Verification items for the finished model (mm, model axes). Face numbers are marked on the shaded views. A direction names the side the tool comes from. Round coordinates to 2 decimals unless told otherwise and drop trailing zeros. Write each loop counter-clockwise with the first axis right and the second up, starting at its lowest first coordinate (ties: lowest second). Pieces come first, ordered by that corner, then holes. Notation, with made-up numbers: (-39, 2) - (-29, 2) arc R10 cw to (-29, 9) - close; hole circle Ø9 at (3, -22.5). An arc over 180 degrees is marked (long way). Answer as a JSON object with one key per item and string values.
Autodesk Inventor part; units mm, degrees
ref_plane "YZ Plane" through (0, 0, 0) normal (1, 0, 0) x (0, 1, 0)
ref_plane "XZ Plane" through (0, 0, 0) normal (0, 1, 0) x (-1, 0, 0)
ref_plane "XY Plane" through (0, 0, 0) normal (0, 0, 1) x (1, 0, 0)
sketch "Sketch1" plane through (0, 0, 0) normal (0, 0, 1) x (1, 0, 0)
  line L0 (-32.1306, 17.7406) -> (444.1194, 17.7406)
  line L1 (444.1194, 17.7406) -> (444.1194, -33.0594)
  line L2 (444.1194, -33.0594) -> (-32.1306, -33.0594)
  line L3 (-32.1306, -33.0594) -> (-32.1306, 17.7406)
  point P0 (0, 0)
  dimension "d0" = 476.25
  dimension "d1" = 50.8
extrude "Extrusion1" add sketch "Sketch1" along normal blind 139.7
sketch "Sketch2" plane through (-32.1306, 17.7406, 0) normal (0, 1, 0) x (1, 0, 0)
  line L0 (0, -139.7) -> (476.25, -139.7)
  line L1 (0, 0) -> (476.25, 0)
  line L2 (0, 0) -> (0, -139.7)
  circle A0 centre (75.1417, -80.645) radius 55.88
  circle A1 centre (225.4419, -80.645) radius 55.88
  circle A2 centre (375.7337, -80.645) radius 55.88
  line L3 (150.2833, 0) -> (150.2833, -139.7)
  line L4 (300.5751, 0) -> (300.5751, -139.7)
  line L5 (450.8669, 0) -> (450.8669, -139.7)
  arc A3 (131.0217, -80.645) -> (150.2833, -114.7129) centre (183.3802, -73.521) ccw
  arc A4 (150.2833, -114.7129) -> (169.5619, -80.645) centre (117.2054, -73.5058) ccw
  arc A5 (281.208, -77.0792) -> (300.5751, -114.6812) centre (333.9413, -73.7073) ccw
  arc A6 (300.5751, -114.6812) -> (319.9683, -77.068) centre (267.2357, -73.6855) ccw
  arc A7 (0, -114.6812) -> (19.2617, -80.645) centre (-33.0921, -73.4855) ccw
  arc A8 (431.6137, -80.645) -> (450.8669, -113.4262) centre (483.7537, -72.0665) ccw
  line L6 (450.8669, 0) -> (476.25, 0)
  line L7 (476.25, 0) -> (476.25, -139.7)
  line L8 (476.25, -139.7) -> (450.8669, -139.7)
  line L9 (450.8669, -139.7) -> (450.8669, 0)
  point P0 (32.1306, 0)
  dimension "d4" = 111.76
  dimension "d5" = 111.76
  dimension "d6" = 111.76
  dimension "d7" = 150.2833
  dimension "d8" = 150.2918
  dimension "d9" = 150.2918
  dimension "d10" = 75.1417
  dimension "d11" = 75.1332
  dimension "d12" = 75.1332
  dimension "d13" = 59.055
extrude "Extrusion2" cut sketch "Sketch2" against normal blind 139.7 contours L2 A7 A0 A3 L3 L0 | L3 A4 A1 A5 L4 L0 | L4 A6 A2 A8 L5 L0 | A0 | L5 L1 L7 L0 | A1 | A2
fillet "Fillet1" radius 2.54 1 edges at (418.7363, -7.6594, 113.4262)
fillet "Fillet2" radius 2.54 1 edges at (268.4445, -7.6594, 114.6812)
fillet "Fillet3" radius 2.54 1 edges at (118.1527, -7.6594, 114.7129)
fillet "Fillet4" radius 2.54 1 edges at (-32.1306, -7.6594, 114.6812)
sketch "Sketch3" plane through (-32.1306, 17.7406, 0) normal (0, 1, 0) x (1, 0, 0)
  arc A0 (148.6129, -113.313) -> (151.9544, -113.3138) centre (150.2841, -111.4003) ccw
  arc A1 (298.8914, -113.2506) -> (302.2598, -113.2517) centre (300.5762, -111.3498) ccw
  line L0 (0, 0) -> (450.8669, 0)
  line L1 (37.0382, 0) -> (113.2382, 0)
  line L2 (113.2382, 0) -> (113.2382, -50.8)
  line L3 (113.2382, -50.8) -> (37.0382, -50.8)
  line L4 (37.0382, -50.8) -> (37.0382, 0)
  line L5 (150.2841, -111.4003) -> (150.2841, 5.0811)
  line L6 (263.53, 0) -> (187.33, 0)
  line L7 (187.33, 0) -> (187.33, -50.8)
  line L8 (187.33, -50.8) -> (263.53, -50.8)
  line L9 (263.53, -50.8) -> (263.53, 0)
  line L10 (75.1382, -50.8) -> (75.1382, 0)
  line L11 (300.5762, -111.3498) -> (300.5762, 0)
  line L12 (337.6224, -50.8) -> (337.6224, 0)
  line L13 (337.6224, 0) -> (413.8224, 0)
  line L14 (413.8224, 0) -> (413.8224, -50.8)
  line L15 (413.8224, -50.8) -> (337.6224, -50.8)
  point P0 (32.1306, 0)
  dimension "d20" = 76.2
  dimension "d21" = 50.8
  dimension "d22" = 0
  dimension "d23" = 38.1
  dimension "d24" = 75.1459
extrude "Extrusion3" cut sketch "Sketch3" against normal blind 25.4
properties part number "swirvy"
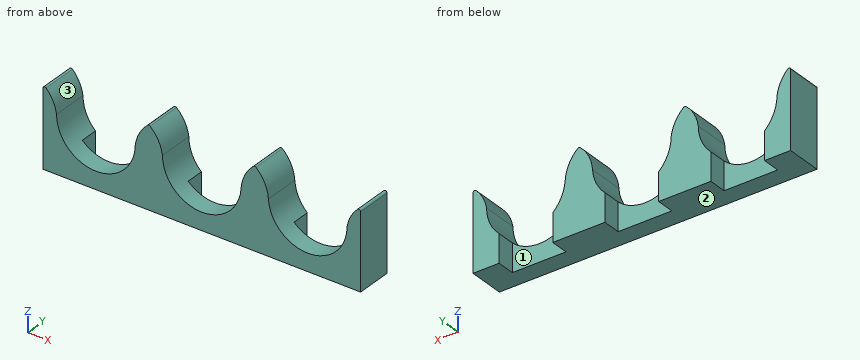
Q1. Material ranges on line 1 along X through (y, z) = (15, 12); line 2 along X through (y, z) = (-19.5, 57); line 3 along Y through (x, z) = (319, 12.5), recorded low to high. Write a range as [from, to].
Geometry check:
{"line 1": "x = [-32.13, 4.91], [81.11, 155.2], [231.4, 305.49], [381.69, 418.74]", "line 2": "x = [-32.13, -7.62], [93.64, 142.68], [243.94, 292.97], [394.23, 418.74]", "line 3": "y = [-33.06, -7.66]"}
Q2. Gauge pin test, flat end, axial feed: P1, Ø20, axis at x = 199.5, z = 11.5, coming from the +Y side. Record the tip position at first contact, or that the pin passes through.
Geometry check:
{"P1": "stops at y = -7.66"}
Q3. Set-up check for the marked faces 1, 2 and 3: record each of +Z, -Z, +X, -X, +Y, -Y from which the full face is reachable in a straight line by a thin tool's end or side.
Geometry check:
{"face 1": "+Z, -Z, +Y", "face 2": "-Z, +X, -X, +Y, -Y", "face 3": "+Z, +Y, -Y"}
Q4. Section check A-A, the plane z = 97.5. Record the cut outline in (x, y).
Geometry check:
{"outline": "(-32.13, -33.06) - (-18.15, -33.06) - (-18.15, 17.74) - (-32.13, 17.74) - close; (104.16, -33.06) - (132.15, -33.06) - (132.15, 17.74) - (104.16, 17.74) - close; (254.63, -33.06) - (282.28, -33.06) - (282.28, 17.74) - (254.63, 17.74) - close; (405.31, -33.06) - (418.74, -33.06) - (418.74, 17.74) - (405.31, 17.74) - close"}
Q5. Section check D-D, the plane z = 51. Record the cut outline in (x, y).
Geometry check:
{"outline": "(-32.13, -33.06) - (-4.36, -33.06) - (-4.36, 17.74) - (-32.13, 17.74) - close; (90.38, -33.06) - (145.94, -33.06) - (145.94, 17.74) - (90.38, 17.74) - close; (240.68, -33.06) - (296.23, -33.06) - (296.23, 17.74) - (240.68, 17.74) - close; (390.97, -33.06) - (418.74, -33.06) - (418.74, 17.74) - (390.97, 17.74) - close"}
Q6. Section check C-C, the plane x = 367.5. Record the cut outline in (y, z), then the cut area to 3 significant figures.
Geometry check:
{"outline": "(-33.06, 0) - (-7.66, 0) - (-7.66, 30.13) - (-33.06, 30.13) - close", "area": "765 mm2"}
Q7. Section check B-B, the plane y = 12. State how many separate pieces and enclosed holes the cut face has, then the cut area to 3 significant figures.
Geometry check:
{"separate pieces": "4", "enclosed holes": "0", "area": "17,400 mm2"}
